from build123d import *

# Parameters (mm, degrees)
EXTRUDE_1_DEPTH   = 2
HOLE_WIZARD_M81_D = 9
CHAMFER_1_SIZE    = 2.5


with BuildPart() as part:
    # Эскиз3 → Бобышка-Вытянуть1 (new body)
    with BuildSketch(Plane(origin=(0, 0, 0), x_dir=(1, 0, 0), z_dir=(0, 0, -1))):
        Polygon((0, 0), (100, 0), (100, 158.205080757), (65.358983849, 178.205080757), (0, 65), align=None)
    extrude(amount=EXTRUDE_1_DEPTH)

    # Отверстие с зазором M81 (through all)
    with Locations(Plane(origin=(0, 0, -2), x_dir=(1, 0, 0), z_dir=(0, 0, -1))):
        with Locations((20, 20), (80, 20), (25, 68.301270189), (72.679491924, 150.884572681)):
            Hole(HOLE_WIZARD_M81_D / 2)

    # Фаска1
    chamfer_1_edges = [part.edges().sort_by_distance(p)[0] for p in [
        (65.358983849, -178.205080757, -1),
        (100, 0, -1),
        (0, 0, -1),
    ]]
    chamfer(chamfer_1_edges, length=CHAMFER_1_SIZE)


solid = part.part
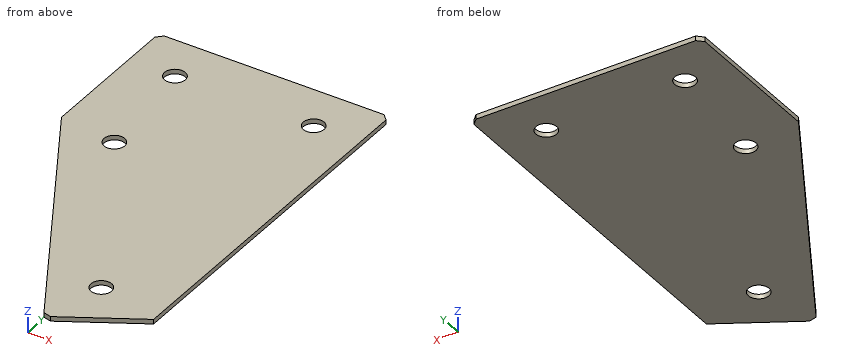
Design review of the part built by this model. Coordinates are the model's own, in mm. Round coordinates to 2 decimals unless told otherwise and drop trailing zeros. Write each loop counter-clockwise with the first axis right and the second up, starting at its lowest first coordinate (ties: lowest second). Pieces come first, ordered by that corner, then holes.
Item 1: Consider section B-B on x = 79. Give the boundary of the cut face in (y, z), and give its area (3 significant figures).
Item 2: Consider section D-D on z = -0.7. Give the boundary of the cut face in (x, y).
Item 3: Consider section A-A on y = -20. Give the boundary of the cut face in (x, z), and give its area (3 significant figures).
Item 4: Wall thickness on L1, parallel to X at y = -20, z = -0.6; L2, parallel to X at y = -21.5, z = -1.4; L3, parallel to Y at x = 24, z = -0.7: over which ranges is each line inside the solid? List them lowest first.
Item 5: Consider section C-C on y = -149. Give the boundary of the cut face in (x, z).
Item 6: For pin 1 Ø1 at (y, z) = (-83, -0.5) entering from -X; pin 2 Ø8 at (x, y) = (25, -68.3) entering from -Z, all flat-tipped, find the tip position at first contact; note any pin that passes through.
Check values:
1. outline: (-170.33, -2) - (-24.39, -2) - (-24.39, 0) - (-170.33, 0) - close; (-15.61, -2) - (0, -2) - (0, 0) - (-15.61, 0) - close
1. area: 323 mm2
2. outline: (0, -65) - (64.11, -176.04) - (67.52, -176.96) - (100, -158.21) - (100, -2.5) - (97.5, 0) - (2.5, 0) - (0, -2.5) - close; hole circle Ø9 at (20, -20); hole circle Ø9 at (25, -68.3); hole circle Ø9 at (72.68, -150.88); hole circle Ø9 at (80, -20)
3. outline: (0, -2) - (15.5, -2) - (15.5, 0) - (0, 0) - close; (24.5, -2) - (75.5, -2) - (75.5, 0) - (24.5, 0) - close; (84.5, -2) - (100, -2) - (100, 0) - (84.5, 0) - close
3. area: 164 mm2
4. L1: x = 0 to 15.5, 24.5 to 75.5, 84.5 to 100
4. L2: x = 0 to 15.76, 24.24 to 75.76, 84.24 to 100
4. L3: y = -106.57 to -72.69, -63.91 to -22.06, -17.94 to 0
5. outline: (48.5, -2) - (68.59, -2) - (68.59, 0) - (48.5, 0) - close; (76.77, -2) - (100, -2) - (100, 0) - (76.77, 0) - close
6. pin 1: stops at x = 10.1
6. pin 2: passes through
